Drawing for the job (mm, zero at the part's lowest x, y, z). A direction names the side the tool comes from. Round coordinates to 2 decimals unless told otherwise and drop trailing zeros. Write each loop counter-clockwise with the first axis right and the second up, starting at its lowest first coordinate (ties: lowest second). Pieces come first, ordered by that corner, then holes. Notation, with made-up numbers: (-9, 2) -> (39, 2) arc R29 cw to (39, 27) -> close; hole circle Ø2 at (-27, 71). An arc over 180 degrees is marked (long way). One line per question, with ' | ' between items.
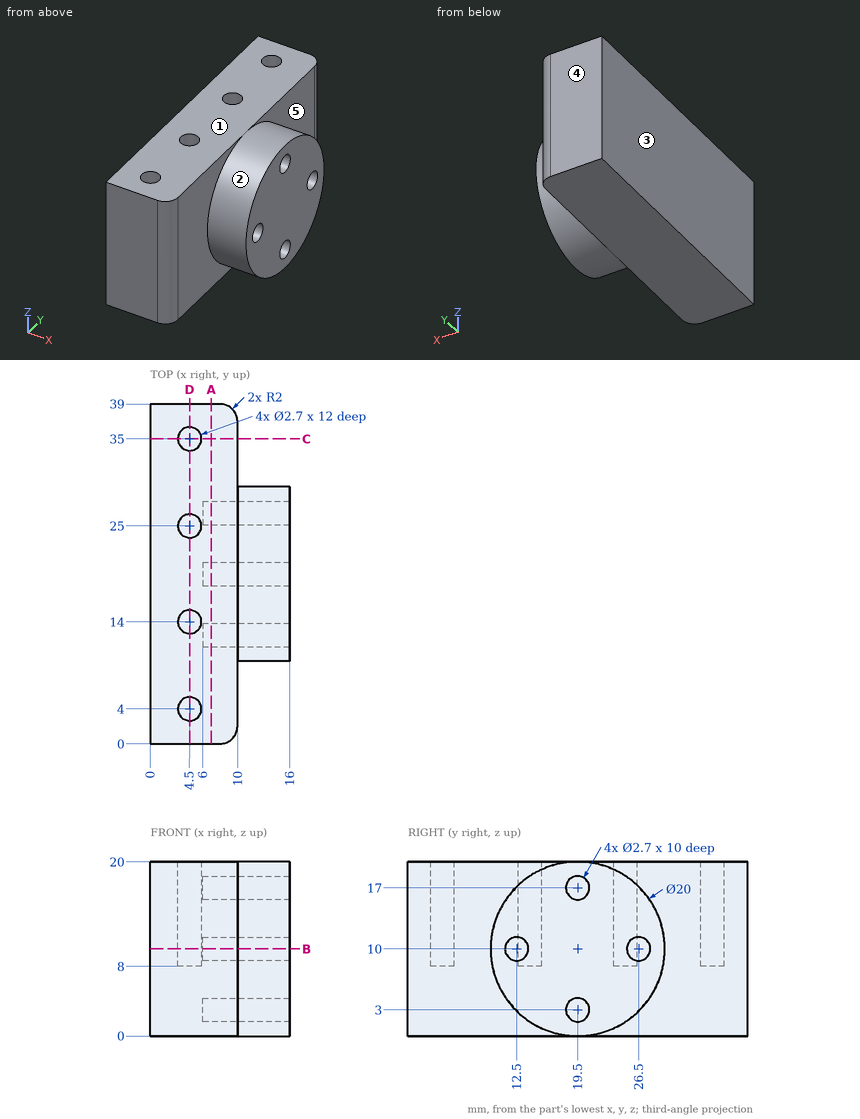
(1) Slice it at A-A (x = 7). Write the cut outline in (y, z), then the cut area to 3 significant figures.
Calculated:
outline: (0, 0) -> (39, 0) -> (39, 20) -> (0, 20) -> close; hole circle Ø2.7 at (12.5, 10); hole circle Ø2.7 at (19.5, 3); hole circle Ø2.7 at (19.5, 17); hole circle Ø2.7 at (26.5, 10) | area: 757 mm2
(2) Mould opens along X. For the marked faces 3, 4 and 5 say: pulls with the +X half, pulls with the -X half, needs draft (parallel to the pull), parting line crosses it, or undercut.
Calculated:
face 3: pulls with the -X half | face 4: needs draft | face 5: pulls with the +X half
(3) Slice it at B-B (z = 10). Write the cut outline in (x, y).
Calculated:
outline: (0, 0) -> (8, 0) arc R2 ccw to (10, 2) -> (10, 9.5) -> (16, 9.5) -> (16, 11.15) -> (6, 11.15) -> (6, 13.85) -> (16, 13.85) -> (16, 25.15) -> (6, 25.15) -> (6, 27.85) -> (16, 27.85) -> (16, 29.5) -> (10, 29.5) -> (10, 37) arc R2 ccw to (8, 39) -> (0, 39) -> close; hole circle Ø2.7 at (4.5, 4); hole circle Ø2.7 at (4.5, 14); hole circle Ø2.7 at (4.5, 25); hole circle Ø2.7 at (4.5, 35)
(4) 3-axis set-ups, long thin cutter, end or side, ignore diameter. For the marked faces 1 and 2: which of +Z, -Z, +X, -X, +Y, -Y reach the whole face in a straight line?
Calculated:
face 1: +Z, +X, -X, +Y, -Y | face 2: +X
(5) Drop flat-ended pins along their axis: pin 1 (1.6 mm diameter, centred on x = 4.5, y = 14, fed in from +Z); pin 2 (5 mm diameter, centred on x = 11.5, z = 11.5, fed in from -Y); pin 3 (1.6 mm diameter, centred on y = 26.5, z = 10, fed in from +X). Give the stop position or say it passes through.
Calculated:
pin 1: z = 8 | pin 2: y = 0.27 | pin 3: x = 6
(6) Slice it at D-D (x = 4.5). Write the cut outline in (y, z), then the cut area to 3 significant figures.
Calculated:
outline: (0, 0) -> (39, 0) -> (39, 20) -> (36.35, 20) -> (36.35, 8) -> (33.65, 8) -> (33.65, 20) -> (26.35, 20) -> (26.35, 8) -> (23.65, 8) -> (23.65, 20) -> (15.35, 20) -> (15.35, 8) -> (12.65, 8) -> (12.65, 20) -> (5.35, 20) -> (5.35, 8) -> (2.65, 8) -> (2.65, 20) -> (0, 20) -> close | area: 650 mm2
(7) Slice it at C-C (y = 35). Write the cut outline in (x, z).
Calculated:
outline: (0, 0) -> (10, 0) -> (10, 20) -> (5.85, 20) -> (5.85, 8) -> (3.15, 8) -> (3.15, 20) -> (0, 20) -> close
(8) Wall check: line 1 (Y direction, x = 4.5, z = 12); line 2 (Y direction, x = 13.25, z = 10); line 3 (Z direction, x = 7.75, y = 19). Give the ranges that are in metal, low to high. Write a range as from..to.
Calculated:
line 1: 0..2.65, 5.35..12.65, 15.35..23.65, 26.35..33.65, 36.35..39 | line 2: 9.5..11.15, 13.85..25.15, 27.85..29.5 | line 3: 0..1.75, 4.25..15.75, 18.25..20
